The model under review builds one solid part; all positions refer to its coordinate system, in mm. Coordinates: 2 decimals unless noted, no trailing zeros. Loops run counter-clockwise (first coordinate to the right, second up) from the corner with the lowest first, then second, coordinate; pieces in that order, holes last. Notation, with made-up numbers: M 60,29 L 69,29 A9 cw 69,40 Z; hole C 46.5,-33.75 d9. An arc over 180 degrees is marked long. Use CSV: the item, a comma, the result in double quotes. Start each with the question number.
1. Add section B-B, the plane z = 1.4. State how many separate pieces and enclosed holes the cut face has, then the cut area to 3 significant figures.
2. Draft analysis for pull direction X (two halves, no side actions). For faces 1 (the flat face through (-0.5, -29, 2)), 2 (the cylindrical face through (-2.5, -33, 2.5)), 3 (the cylindrical face through (0, 45, 2)), state which applies: +X half, -X half, draft (parallel to the pull), parting line (faces both ways), or undercut.
3. Clearance check with flat-ended pins moving along their axes: P1, Ø1, axis at x = -15, z = 2, coming from the +Y side; P2, Ø1.7, axis at x = -23, z = 2.5, coming from the -Y side; P3, Ø1, axis at y = -14.5, z = 2.5, coming from the -X side; P4, Ø6, axis at x = -3, y = 13.5, coming from the -Z side. State where each tip first meets the part, or that it passes through.
4. Add section A-A, the plane x = 8.5. Write out the cut boundary in (y, z).
5. For L1, parallel to X at y = 22, z = 1.2; L2, parallel to X at y = -17, z = 0.3; L3, parallel to X at y = 28.5, z = 2.6, list the stretches that pass through material, from the lowest coordinate up.
from build123d import *

# Parameters (mm, degrees)
F0_R     = 1.5
F1_DEPTH = 5
F2_COUNT = 4


with BuildPart() as f1:
    # F0 (on Top) → F1 (new body)
    with BuildSketch(Plane.XY):
        with BuildLine():
            ThreePointArc((-21, 0), (-24.5147186258, 8.4852813742), (-33, 12))
            ThreePointArc((-33, 12), (-44.9999119071, -0.0459806707), (-32.9080393338, -11.9996476297))
            ThreePointArc((-32.9080393338, -11.9996476297), (-24.4822676728, -8.4527058391), (-21, 0))
        make_face()
        Polygon((-21.6812912544, 0.6075373587), (-21.6812912544, 0), (-21.6812912544, -0.4327508824), (-23.7081500818, -0.4327508824), (-23.7081500818, -1.9761508169), (-21.5306197837, -1.9761508169), (-21.5306197837, -3.0243001782), (-24.9777209956, -3.0243001782), (-24.9777209956, 0), (-24.9777209956, 2.9619428615), (-21.5306197837, 2.9619428615), (-21.5306197837, 1.9216546204), (-23.7081500818, 1.9216546204), (-23.7081500818, 0.6075373587), align=None, mode=Mode.SUBTRACT)
        with BuildLine():
            ThreePointArc((-27.0208696284, 0.5), (-27.0052196775, 0.2502176759), (-27, 0))
            ThreePointArc((-27, 0), (-27.0052196775, -0.2502176759), (-27.0208696284, -0.5))
            ThreePointArc((-27.0208696284, -0.5), (-33, -6), (-38.9791303716, -0.5))
            ThreePointArc((-38.9791303716, -0.5), (-39, 0), (-38.9791303716, 0.5))
            ThreePointArc((-38.9791303716, 0.5), (-33, 6), (-27.0208696284, 0.5))
        make_face(mode=Mode.SUBTRACT)
        with BuildLine():
            ThreePointArc((-11, 0), (-7.7781745931, 7.7781745931), (0, 11))
            Line((0, 11), (0, 12))
            Line((0, 12), (-33, 12))
            ThreePointArc((-33, 12), (-24.5147186258, 8.4852813742), (-21, 0))
            Line((-21, 0), (-20.2820118571, 0))
            Line((-20.2820118571, 0), (-20.2820118571, 2.9619428615))
            Line((-20.2820118571, 2.9619428615), (-19.0124409432, 2.9619428615))
            Line((-19.0124409432, 2.9619428615), (-19.0124409432, 0))
            Line((-19.0124409432, 0), (-15.5443767441, 0))
            Line((-15.5443767441, 0), (-15.5443767441, 2.9619428615))
            Line((-15.5443767441, 2.9619428615), (-14.2748058302, 2.9619428615))
            Line((-14.2748058302, 2.9619428615), (-14.2748058302, 0))
            Line((-14.2748058302, 0), (-11, 0))
        make_face()
        with BuildLine():
            Line((0, -11.9996476297), (0, -11))
            ThreePointArc((0, -11), (-7.7781745931, -7.7781745931), (-11, 0))
            Line((-11, 0), (-14.2748058302, 0))
            Line((-14.2748058302, 0), (-14.2748058302, -3.0243001782))
            Line((-14.2748058302, -3.0243001782), (-15.5443767441, -3.0243001782))
            Line((-15.5443767441, -3.0243001782), (-15.5443767441, 0))
            Line((-15.5443767441, 0), (-19.0124409432, 0))
            Line((-19.0124409432, 0), (-19.0124409432, -1.9761508169))
            Line((-19.0124409432, -1.9761508169), (-16.5846649851, -1.9761508169))
            Line((-16.5846649851, -1.9761508169), (-16.5846649851, -3.0243001782))
            Line((-16.5846649851, -3.0243001782), (-20.2820118571, -3.0243001782))
            Line((-20.2820118571, -3.0243001782), (-20.2820118571, 0))
            Line((-20.2820118571, 0), (-21, 0))
            ThreePointArc((-21, 0), (-24.4822676728, -8.4527058391), (-32.9080393338, -11.9996476297))
            Line((-32.9080393338, -11.9996476297), (0, -11.9996476297))
        make_face()
        with BuildLine():
            ThreePointArc((-30.5505102572, -0.5), (-30.5126596175, -0.251272405), (-30.5, 0))
            ThreePointArc((-30.5, 0), (-30.5126596175, 0.251272405), (-30.5505102572, 0.5))
            ThreePointArc((-30.5505102572, 0.5), (-33, 2.5), (-35.4494897428, 0.5))
            ThreePointArc((-35.4494897428, 0.5), (-35.5, 0), (-35.4494897428, -0.5))
            ThreePointArc((-35.4494897428, -0.5), (-33, -2.5), (-30.5505102572, -0.5))
        make_face()
        with Locations((-33, 0)):
            Circle(F0_R, mode=Mode.SUBTRACT)
        with BuildLine():
            Line((-35.4494897428, 0.5), (-38.9791303716, 0.5))
            ThreePointArc((-38.9791303716, 0.5), (-39, 0), (-38.9791303716, -0.5))
            Line((-38.9791303716, -0.5), (-35.4494897428, -0.5))
            ThreePointArc((-35.4494897428, -0.5), (-35.5, 0), (-35.4494897428, 0.5))
        make_face()
        with BuildLine():
            ThreePointArc((-27.0208696284, -0.5), (-27.0052196775, -0.2502176759), (-27, 0))
            Line((-27, 0), (-30.5, 0))
            ThreePointArc((-30.5, 0), (-30.5126596175, -0.251272405), (-30.5505102572, -0.5))
            Line((-30.5505102572, -0.5), (-27.0208696284, -0.5))
        make_face()
        with BuildLine():
            Line((-30.5, 0), (-27, 0))
            ThreePointArc((-27, 0), (-27.0052196775, 0.2502176759), (-27.0208696284, 0.5))
            Line((-27.0208696284, 0.5), (-30.5505102572, 0.5))
            ThreePointArc((-30.5505102572, 0.5), (-30.5126596175, 0.251272405), (-30.5, 0))
        make_face()
    extrude(amount=F1_DEPTH)

    # F2: F1 ×4 about axis
    f2_axis = Axis((0, 0, 5), (0, 0, -1))


with BuildPart() as f1_1:
    add(f1.part)
    for i in range(1, F2_COUNT):
        add(f1.part.rotate(f2_axis, i * 360 / F2_COUNT))


solid = f1_1.part
Computed:
1,separate pieces,"1"
1,enclosed holes,"25"
1,area,"2,610 mm^2"
2,face 1,"undercut"
2,face 2,"undercut"
2,face 3,"parting line"
3,P1,"stops at y = 12"
3,P2,"stops at y = -12"
3,P3,"stops at x = -12"
3,P4,"stops at z = 0"
4,outline,"M -41.47,0 L -6.98,0 L -6.98,5 L -41.47,5 Z; M 6.98,0 L 41.47,0 L 41.47,5 L 6.98,5 Z"
5,L1,"x = -12 to -3.02, -1.98 to -0.43, 0.61 to 1.92, 2.96 to 12"
5,L2,"x = -12 to 1.98, 3.02 to 12"
5,L3,"x = -12 to -3.97, -0.5 to 0.5, 3.97 to 12"
